Part model, mm, in its own coordinate system. Give positions to 0.01 mm unless a question says otherwise; leave off trailing zeros. Order: outer loops, then holes, each group sorted by start corner. A loop starts at its lowest first (then second) coordinate and runs counter-clockwise, first axis right, second up.
1. Slice it at C-C on y = 116.5. List the corners of the cut face in (x, z), and give its area (3 significant figures).
2. Slice it at B-B on x = 33.5. List the corners of the cut face in (y, z), and give its area (3 significant figures).
3. Slice it at D-D on z = 1.8. Give the number of separate pieces and of enclosed holes in the cut face, and give its area (3 significant figures).
4. Probe line 1 (Y direction, x = 33.5, z = 1.85); line 2 (Y direction, x = 29, z = 1.5); line 3 (X direction, y = 113, z = 1.5). List the from-to ranges inside material, lowest first.
5. Slice it at A-A on y = -8. List the corners of the cut face in (x, z).
6. Drop flat-ended pins along their axis: pin 1 Ø1 at (x, z) = (0.5, 2) entering from -Y (3 decimals); pin 2 Ø10 at (x, y) = (26, 6.5) entering from -Z; pin 3 Ø1.3 at (y, z) = (39, 2.5) entering from -X; pin 4 Ø0.5 at (x, z) = (4.5, 2.5) entering from -Y (3 decimals). Give the stop position or say it passes through.
from build123d import *

# Parameters (mm, degrees)
SKETCH2_W           = 12.7
SKETCH2_H           = 22.225
BOSS_EXTRUDE2_DEPTH = 4.2926
BOSS_EXTRUDE3_DEPTH = 4.2926
SKETCH5_W           = 4.2926
SKETCH5_H           = 31.75
CUT_EXTRUDE2_DEPTH  = 4.2926
SKETCH6_W           = 4.2926
SKETCH6_H           = 38.1
CUT_EXTRUDE3_DEPTH  = 4.2926
SKETCH9_W           = 4.2926
SKETCH9_H           = 44.45
BOSS_EXTRUDE4_DEPTH = 6.35
SKETCH10_W          = 4.2926
SKETCH10_H          = 6.35
BOSS_EXTRUDE5_DEPTH = 6.35
SKETCH12_W          = 4.2926
SKETCH12_H          = 44.45
BOSS_EXTRUDE6_DEPTH = 8.382
FILLET4_R           = 1.27
CUT_EXTRUDE1_DEPTH  = 4.2926


with BuildPart() as part:
    # Sketch2 → Boss-Extrude2 (new body)
    with BuildSketch(Plane.XY):
        Polygon((6.35, 48.384354874), (6.35, 101.6), (-6.35, 101.6), (-6.35, 48.384354874), (-6.35, 22.225), (6.35, 22.225), align=None)
        with Locations((0, 11.1125)):
            Rectangle(SKETCH2_W, SKETCH2_H)
        Polygon((10.541, 22.225), (6.35, 22.225), (6.35, 0), (-6.35, 0), (-6.35, 22.225), (-10.541, 22.225), (-10.541, -22.225), (10.541, -22.225), align=None)
        Polygon((6.35, 156.723399657), (6.35, 101.6), (6.35, 48.384354874), (84.403334241, 48.384354874), align=None)
        Polygon((-6.35, 101.6), (6.35, 101.6), (6.35, 156.723399657), (-47.828182898, 48.384354874), (-6.35, 48.384354874), align=None)
    extrude(amount=BOSS_EXTRUDE2_DEPTH)

    # Sketch2_3 → Boss-Extrude3 (add)
    with BuildSketch(Plane.XY):
        Polygon((-6.35, 101.6), (6.35, 101.6), (6.35, 156.723399657), (-47.828182898, 48.384354874), (-6.35, 48.384354874), align=None)
    extrude(amount=BOSS_EXTRUDE3_DEPTH)

    # Sketch5 → Cut-Extrude2 (cut)
    with BuildSketch(Plane(origin=(0, 0, 0), x_dir=(-1, 0, 0), z_dir=(0, 0, -1))):
        with Locations((0, -6.35)):
            Rectangle(SKETCH5_W, SKETCH5_H)
    extrude(amount=-CUT_EXTRUDE2_DEPTH, mode=Mode.SUBTRACT)

    # Sketch6 → Cut-Extrude3 (cut)
    with BuildSketch(Plane(origin=(0, 0, 0), x_dir=(-1, 0, 0), z_dir=(0, 0, -1))):
        with Locations((-4.2926, -3.175)):
            Rectangle(SKETCH6_W, SKETCH6_H)
    extrude(amount=-CUT_EXTRUDE3_DEPTH, mode=Mode.SUBTRACT)

    # Sketch9 → Boss-Extrude4 (add)
    with BuildSketch(Plane(origin=(10.541, 0, 0), x_dir=(0, 0, -1), z_dir=(1, 0, 0))):
        with Locations((-2.1463, 0)):
            Rectangle(SKETCH9_W, SKETCH9_H)
    extrude(amount=BOSS_EXTRUDE4_DEPTH)

    # Sketch10 → Boss-Extrude5 (add)
    with BuildSketch(Plane(origin=(6.35, 0, 0), x_dir=(0, 0, -1), z_dir=(1, 0, 0))):
        with Locations((-2.1463, 25.4)):
            Rectangle(SKETCH10_W, SKETCH10_H)
    extrude(amount=BOSS_EXTRUDE5_DEPTH)

    # Sketch12 → Boss-Extrude6 (add)
    with BuildSketch(Plane.ZY.offset(10.541)):
        with Locations((2.1463, 0)):
            Rectangle(SKETCH12_W, SKETCH12_H)
    extrude(amount=BOSS_EXTRUDE6_DEPTH)

    # Fillet4
    fillet4_edges = [part.edges().sort_by_distance(p)[0] for p in [
        (2.1463, 15.875, 2.1463),
        (6.4389, -22.225, 2.1463),
        (6.4389, 15.875, 2.1463),
        (16.891, -22.225, 2.1463),
        (16.891, 22.225, 2.1463),
        (6.35, 28.575, 2.1463),
        (12.7, 28.575, 2.1463),
        (-18.923, -22.225, 2.1463),
        (-18.923, 22.225, 2.1463),
        (-6.35, 22.225, 2.1463),
        (-47.828182898, 48.384354874, 2.1463),
        (6.35, 156.723399657, 2.1463),
        (84.403334241, 48.384354874, 2.1463),
        (-2.1463, 9.525, 2.1463),
        (-2.1463, -22.225, 2.1463),
        (2.1463, 9.525, 2.1463),
    ]]
    fillet(fillet4_edges, radius=FILLET4_R)

    # Sketch4 → Cut-Extrude1 (cut)
    with BuildSketch(Plane(origin=(0, 0, 0), x_dir=(-1, 0, 0), z_dir=(0, 0, -1))):
        Polygon((-2.761203873, 129.144568559), (-1.308492387, 96.220137091), (25.689356606, 71.698449698), align=None)
        Polygon((-12.368070704, 129.144568559), (-16.525699657, 95.623732399), (-57.420105949, 62.352675196), align=None)
        Polygon((-7.819762817, 87.308153563), (-45.531165478, 59.983677251), (20.045786345, 61.339421803), align=None)
    extrude(amount=-CUT_EXTRUDE1_DEPTH, mode=Mode.SUBTRACT)


solid = part.part
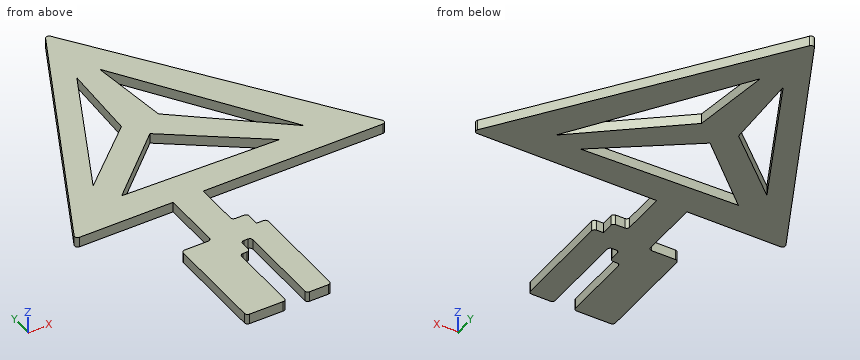
Data:
1. outline: (-13.76, 0) - (-3.5, 0) - (-3.5, 4.29) - (-13.76, 4.29) - close; (2.2, 0) - (13.94, 0) - (13.94, 4.29) - (2.2, 4.29) - close; (20.9, 0) - (35.33, 0) - (35.33, 4.29) - (20.9, 4.29) - close
1. area: 156 mm2
2. outline: (48.38, 0) - (60.23, 0) - (60.23, 4.29) - (48.38, 4.29) - close; (68.7, 0) - (81.81, 0) - (81.81, 4.29) - (68.7, 4.29) - close; (97.82, 0) - (119.04, 0) - (119.04, 4.29) - (97.82, 4.29) - close
2. area: 198 mm2
3. separate pieces: 1
3. enclosed holes: 3
3. area: 6,910 mm2
4. line 1: y = 48.38 to 60.23, 68.7 to 81.81, 97.82 to 119.04
4. line 2: y = 48.38 to 60.33, 71.96 to 85.47, 104.49 to 125.28
4. line 3: x = -15.52 to -5.23, 2.05 to 14.37, 23.26 to 37.85
5. outline: (-18.92, 0) - (-2.15, 0) - (-2.15, 4.29) - (-18.92, 4.29) - close; (6.44, 0) - (16.89, 0) - (16.89, 4.29) - (6.44, 4.29) - close
6. pin 1: stops at y = 9.525
6. pin 2: passes through
6. pin 3: stops at x = -6.35
6. pin 4: stops at y = 15.875
